from build123d import *

# Parameters (mm, degrees)
SKETCH1_W                       = 96
SKETCH1_H                       = 96
BOSS_EXTRUDE1_DEPTH             = 8
SKETCH2_W                       = 92
SKETCH2_H                       = 92
COMPONENT_PLATFORM_DEPTH        = 6
CABLE_SLOTS_DEPTH               = 6
SKETCH4_R                       = 7.5
CENTER_MASS_CUT_DEPTH           = 6
INNER_CORNER_FILLETS_R          = 3
TAP_DRILL_FOR_M3X0_5_TAP4_D     = 2.5
TAP_DRILL_FOR_M3X0_5_TAP4_DEPTH = 2
TAP_DRILL_FOR_M2X0_4_TAP2_D     = 1.6
TAP_DRILL_FOR_M2X0_4_TAP1_D     = 1.6
TAP_DRILL_FOR_M2X0_4_TAP1_DEPTH = 2
CUT_EXTRUDE1_START              = -8
SKETCH28_OUTSIDE_W              = 125.2
SKETCH28_OUTSIDE_H              = 125.2
SKETCH28_OUTSIDE_W_2            = 95
SKETCH28_OUTSIDE_H_2            = 95
CUT_EXTRUDE1_DEPTH              = 8


with BuildPart() as part:
    # Sketch1 → Boss-Extrude1 (new body)
    with BuildSketch(Plane.XY):
        Rectangle(SKETCH1_W, SKETCH1_H)
    extrude(amount=BOSS_EXTRUDE1_DEPTH)

    # Sketch2 → Component Platform (cut)
    with BuildSketch(Plane.XY.offset(8)):
        Rectangle(SKETCH2_W, SKETCH2_H)
    extrude(amount=-COMPONENT_PLATFORM_DEPTH, mode=Mode.SUBTRACT)

    # Sketch3 → Cable Slots (cut, symmetric)
    with BuildSketch(Plane.XY.offset(2)):
        with BuildLine():
            Line((-40.878679656, -25.121320344), (-33.878679656, -18.121320344))
            ThreePointArc((-33.878679656, -18.121320344), (-33.228361402, -17.148050297), (-33, -16))
            Line((-33, -16), (-33, 16))
            ThreePointArc((-33, 16), (-33.228361402, 17.148050297), (-33.878679656, 18.121320344))
            Line((-33.878679656, 18.121320344), (-40.878679656, 25.121320344))
            ThreePointArc((-40.878679656, 25.121320344), (-41.851949703, 25.771638598), (-43, 26))
            Line((-43, 26), (-48, 26))
            Line((-48, 26), (-48, -26))
            Line((-48, -26), (-43, -26))
            ThreePointArc((-43, -26), (-41.851949703, -25.771638598), (-40.878679656, -25.121320344))
        make_face()
        with BuildLine():
            Line((48, -26), (48, 26))
            Line((48, 26), (43, 26))
            ThreePointArc((43, 26), (41.851949703, 25.771638598), (40.878679656, 25.121320344))
            Line((40.878679656, 25.121320344), (33.878679656, 18.121320344))
            ThreePointArc((33.878679656, 18.121320344), (33.228361402, 17.148050297), (33, 16))
            Line((33, 16), (33, -16))
            ThreePointArc((33, -16), (33.228361402, -17.148050297), (33.878679656, -18.121320344))
            Line((33.878679656, -18.121320344), (40.878679656, -25.121320344))
            ThreePointArc((40.878679656, -25.121320344), (41.851949703, -25.771638598), (43, -26))
            Line((43, -26), (48, -26))
        make_face()
    extrude(amount=CABLE_SLOTS_DEPTH, both=True, mode=Mode.SUBTRACT)

    # Sketch4 → Center Mass Cut (cut)
    with BuildSketch(Plane.XY.offset(2)):
        Circle(SKETCH4_R)
    extrude(amount=-CENTER_MASS_CUT_DEPTH, mode=Mode.SUBTRACT)

    # Inner Corner Fillets
    inner_corner_fillets_edges = [part.edges().sort_by_distance(p)[0] for p in [
        (-46, -46, 5),
        (-46, 46, 5),
        (46, 46, 5),
        (46, -46, 5),
    ]]
    fillet(inner_corner_fillets_edges, radius=INNER_CORNER_FILLETS_R)

    # Tap Drill for M3x0.5 Tap4
    with Locations(Plane(origin=(0, -48, 0), x_dir=(-1, 0, 0), z_dir=(0, -1, 0))):
        with Locations((35, -5), (-35, -5)):
            tap_drill_for_m3x0_5_tap4 = Hole(TAP_DRILL_FOR_M3X0_5_TAP4_D / 2, depth=TAP_DRILL_FOR_M3X0_5_TAP4_DEPTH)

    # Mirror2: Tap Drill for M3x0.5 Tap4 across plane
    add(tap_drill_for_m3x0_5_tap4.mirror(Plane(origin=(0, 0, 0), x_dir=(0, 0, 1), z_dir=(0, -1, 0))), mode=Mode.SUBTRACT)

    # Tap Drill for M2x0.4 Tap2 (through all)
    with Locations(Plane.XY.offset(2)):
        with Locations((-17.3, 36.05), (-17.3, 24.85), (-17.3, 15.45), (-17.3, 4.05), (17.3, 4.05), (17.3, 15.45), (17.3, 24.85), (17.3, 36.05), (17.3, -4.75), (17.3, -15.75), (17.3, -25.45), (17.3, -36.05), (-17.3, -4.75), (-17.3, -15.75), (-17.3, -25.45), (-17.3, -36.05)):
            Hole(TAP_DRILL_FOR_M2X0_4_TAP2_D / 2)

    # Tap Drill for M2x0.4 Tap1
    with Locations(Plane(origin=(48, 0, 0), x_dir=(0, 0, -1), z_dir=(1, 0, 0))):
        with Locations((-5, -35), (-5, 35)):
            tap_drill_for_m2x0_4_tap1 = Hole(TAP_DRILL_FOR_M2X0_4_TAP1_D / 2, depth=TAP_DRILL_FOR_M2X0_4_TAP1_DEPTH)

    # Mirror3: Tap Drill for M2x0.4 Tap1 across plane
    add(tap_drill_for_m2x0_4_tap1.mirror(Plane(origin=(0, 0, 0), x_dir=(0, 0, 1), z_dir=(1, 0, 0))), mode=Mode.SUBTRACT)

    # Sketch28 outside → Cut-Extrude1 (cut)
    with BuildSketch(Plane(origin=(0, 0, 0), x_dir=(-1, 0, 0), z_dir=(0, 0, -1)).offset(CUT_EXTRUDE1_START)):
        Rectangle(SKETCH28_OUTSIDE_W, SKETCH28_OUTSIDE_H)
        Rectangle(SKETCH28_OUTSIDE_W_2, SKETCH28_OUTSIDE_H_2, mode=Mode.SUBTRACT)
    extrude(amount=CUT_EXTRUDE1_DEPTH, mode=Mode.SUBTRACT)


solid = part.part
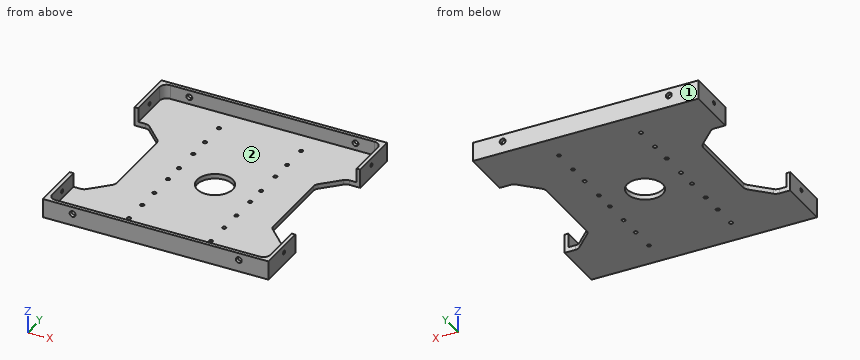
Can you work these out from the model? Positions are in its coordinate system, mm. Face numbers are marked on the shaded views. Round coordinates to 2 decimals unless told otherwise and drop trailing zeros. Write each loop counter-clockwise with the first axis right and the second up, starting at its lowest first coordinate (ties: lowest second). Pieces come first, ordered by that corner, then holes. Notation, with made-up numbers: M 15.25,-40 L 64.25,-40 A21 cw 64.25,-22 Z; hole C 51,-14 d1. An arc over 180 degrees is marked long. Use a Markdown table: item, result.
Item 1: For pin 1 Ø2 at (y, z) = (8, 0.5) entering from +X; pin 2 Ø17 at (x, y) = (0, 0) entering from +Z; pin 3 Ø1.3 at (x, y) = (-17.3, -15.75) entering from -Z; pin 4 Ø1.6 at (y, z) = (1.5, 0.5) entering from -X, each with a flat end and sliding along its axis, tell me the tip position at first contact or that it passes through.
Found:
| item | result |
|---|---|
| pin 1 | stops at x = 33 |
| pin 2 | stops at z = 2 |
| pin 3 | passes through |
| pin 4 | stops at x = -33 |
Item 2: We'd pull the mould along X, two halves only. Please class the marked faces 1 and 2: released by +X, released by -X, zero draft, split by the parting line, or undercut.
Found:
| item | result |
|---|---|
| face 1 | zero draft |
| face 2 | undercut |
Item 3: I want a section at B-B (y = 0). List the corners of the cut face in (x, z) for me.
Found:
| item | result |
|---|---|
| outline | M -33,0 L -7.5,0 L -7.5,2 L -33,2 Z; M 7.5,0 L 33,0 L 33,2 L 7.5,2 Z |
Item 4: I want a section at C-C (y = -31). List the corners of the cut face in (x, z) for me.
Found:
| item | result |
|---|---|
| outline | M -47.5,0 L 47.5,0 L 47.5,8 L 46,8 L 46,2 L -46,2 L -46,8 L -47.5,8 Z |
Item 5: I want a section at A-A (x = 0). List the corners of the cut face in (y, z) for me.
Found:
| item | result |
|---|---|
| outline | M -47.5,0 L -7.5,0 L -7.5,2 L -46,2 L -46,8 L -47.5,8 Z; M 7.5,0 L 47.5,0 L 47.5,8 L 46,8 L 46,2 L 7.5,2 Z |
Item 6: If I drill on line 1 along Y through (x, z) = (46.45, 5); line 2 along X through (y, z) = (-46.65, 5); line 3 along X through (y, z) = (-43, 5), over which ranges is the centre line in solid material (lowest first)? Write a range as [from, to].
Found:
| item | result |
|---|---|
| line 1 | y = [-47.5, -35.8], [-34.2, -26], [26, 34.2], [35.8, 47.5] |
| line 2 | x = [-47.5, -36.25], [-33.75, 33.75], [36.25, 47.5] |
| line 3 | x = [-47.5, -46], [46, 47.5] |
